from build123d import *

# Parameters (mm, degrees)
SKETCH1_W                       = 66
SKETCH1_H                       = 95
CRADLE_BASE_DEPTH               = 3
SKETCH2_R                       = 3
STANDOFFS_DEPTH                 = 10
PILOT_AND_BOLT_HOLES_DEPTH      = 144.412865532
PILOT_AND_BOLT_HOLES_DEPTH_BACK = 144.412865532
SKETCH3_R                       = 1.1
SKETCH3_R_2                     = 1.7
USB_END_NOTCH_DEPTH             = 144.412865532
USB_END_NOTCH_DEPTH_BACK        = 144.412865532
SKETCH4_W                       = 8
SKETCH4_H                       = 4


with BuildPart() as part:
    # Sketch1 → Cradle Base (new body)
    with BuildSketch(Plane(origin=(0, 0, 0), x_dir=(1, 0, 0), z_dir=(0, 1, 0))):
        with Locations((-98, 10)):
            Rectangle(SKETCH1_W, SKETCH1_H)
    extrude(amount=-CRADLE_BASE_DEPTH)

    # Sketch2 → Standoffs (add)
    with BuildSketch(Plane(origin=(0, 0, 0), x_dir=(1, 0, 0), z_dir=(0, 1, 0))):
        with Locations(Location((-122.5, 49, 0), (0, 0, 270))):
            Circle(SKETCH2_R)
        with Locations(Location((-122.5, -9, 0), (0, 0, 270))):
            Circle(SKETCH2_R)
        with Locations(Location((-73.5, 49, 0), (0, 0, 270))):
            Circle(SKETCH2_R)
        with Locations(Location((-73.5, -9, 0), (0, 0, 270))):
            Circle(SKETCH2_R)
    extrude(amount=-STANDOFFS_DEPTH)

    # Sketch3 → Pilot and Bolt Holes (cut, two sides: drawn at the far end of the back side and taken through both)
    with BuildSketch(Plane(origin=(0, 0, 0), x_dir=(1, 0, 0), z_dir=(0, 1, 0)).offset(-PILOT_AND_BOLT_HOLES_DEPTH_BACK)):
        with Locations(Location((-122.5, 49, 0), (0, 0, 270))):
            Circle(SKETCH3_R)
        with Locations(Location((-122.5, -9, 0), (0, 0, 270))):
            Circle(SKETCH3_R)
        with Locations(Location((-73.5, 49, 0), (0, 0, 270))):
            Circle(SKETCH3_R)
        with Locations(Location((-73.5, -9, 0), (0, 0, 270))):
            Circle(SKETCH3_R)
        with Locations(Location((-110, -12, 0), (0, 0, 270))):
            Circle(SKETCH3_R_2)
        with Locations(Location((-110, 12, 0), (0, 0, 270))):
            Circle(SKETCH3_R_2)
        with Locations(Location((-86, -12, 0), (0, 0, 270))):
            Circle(SKETCH3_R_2)
        with Locations(Location((-86, 12, 0), (0, 0, 270))):
            Circle(SKETCH3_R_2)
    extrude(amount=PILOT_AND_BOLT_HOLES_DEPTH + PILOT_AND_BOLT_HOLES_DEPTH_BACK, mode=Mode.SUBTRACT)

    # Sketch4 → USB End Notch (cut, two sides: drawn at the far end of the back side and taken through both)
    with BuildSketch(Plane(origin=(0, 0, 0), x_dir=(1, 0, 0), z_dir=(0, 1, 0)).offset(-USB_END_NOTCH_DEPTH_BACK)):
        with Locations((-98, -36.5)):
            Rectangle(SKETCH4_W, SKETCH4_H)
    extrude(amount=USB_END_NOTCH_DEPTH + USB_END_NOTCH_DEPTH_BACK, mode=Mode.SUBTRACT)


solid = part.part
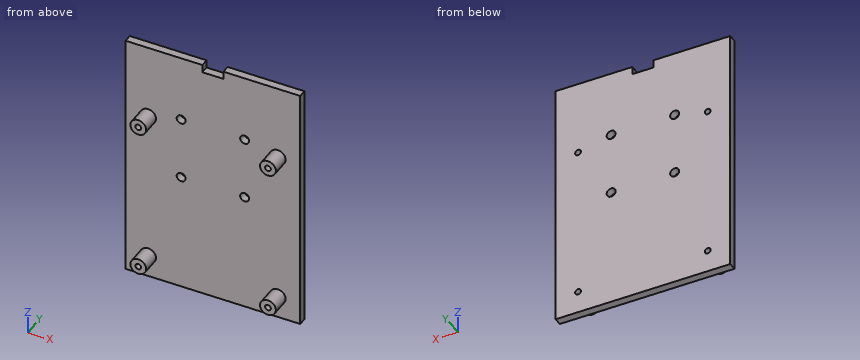
Input: part model. Units: mm. Frame: model coordinates. Give positions to 0.01 mm unless a question says otherwise; leave off trailing zeros. Write each loop counter-clockwise with the first axis right and the second up, starting at its lowest first coordinate (ties: lowest second). Pieces come first, ordered by that corner, then holes. Notation, with made-up numbers: M 65,73 L 87,73 A4 cw 87,77 Z; hole C 17,74.25 d9. An arc over 180 degrees is marked long. Write item = value, one per line. Start each with the question number.
1) Material intervals for line 1 along X through (y, z) = (-8, -49); line 2 along X through (y, z) = (-2.1, -12); line 3 along Z through (x, y) = (-86, -1.35), sorted ascending. Write a range as [from, to].
2) Cut plane B-B on x = -86. Return the cut outline in (y, z), then the cut area to 3 significant figures.
3) Cut plane D-D on x = -122.5. Return the cut outline in (y, z), then the cut area to 3 significant figures.
4) Cut plane A-A on y = -4.5. Return the cut outline in (x, z), then the cut area to 3 significant figures.
5) Cut plane C-C on z = 9. Return the cut outline in (x, y), then the cut area to 3 significant figures.
6) First-contact query: pin 1 Ø20 at (x, z) = (-90.5, 4.5) entering from -Y; pin 2 Ø3.5 at (x, y) = (-97.5, -2) entering from +Z. Flat tips, straight axial feed; report the tip coordinate or a pass-through.
Solved:
q1.line_1 = [-125.5, -123.6], [-121.4, -119.5], [-76.5, -74.6], [-72.4, -70.5]
q1.line_2 = [-131, -111.7], [-108.3, -87.7], [-84.3, -65]
q1.line_3 = [-57.5, -13.7], [-10.3, 10.3], [13.7, 37.5]
q2.outline = M -3,-57.5 L 0,-57.5 L 0,-13.7 L -3,-13.7 Z; M -3,-10.3 L 0,-10.3 L 0,10.3 L -3,10.3 Z; M -3,13.7 L 0,13.7 L 0,37.5 L -3,37.5 Z
q2.area = 265 mm2
q3.outline = M -10,-52 L -3,-52 L -3,-57.5 L 0,-57.5 L 0,-50.1 L -10,-50.1 Z; M -10,-47.9 L 0,-47.9 L 0,7.9 L -10,7.9 L -10,6 L -3,6 L -3,-46 L -10,-46 Z; M -10,10.1 L 0,10.1 L 0,37.5 L -3,37.5 L -3,12 L -10,12 Z
q3.area = 325 mm2
q4.outline = C -122.5,-49 d6; C -122.5,9 d6; C -73.5,-49 d6; C -73.5,9 d6; hole C -122.5,-49 d2.2; hole C -122.5,9 d2.2; hole C -73.5,-49 d2.2; hole C -73.5,9 d2.2
q4.area = 97.9 mm2
q5.outline = M -131,-3 L -125.5,-3 L -125.5,-10 L -123.6,-10 L -123.6,0 L -131,0 Z; M -121.4,-10 L -119.5,-10 L -119.5,-3 L -76.5,-3 L -76.5,-10 L -74.6,-10 L -74.6,0 L -121.4,0 Z; M -72.4,-10 L -70.5,-10 L -70.5,-3 L -65,-3 L -65,0 L -72.4,0 Z
q5.area = 238 mm2
q6.pin_1 = -3
q6.pin_2 = 34.5
